Geometry check sheet. Reference: the model listing, model coordinates, mm. Round coordinates to 2 decimals unless told otherwise and drop trailing zeros. Write each loop counter-clockwise with the first axis right and the second up, starting at its lowest first coordinate (ties: lowest second). Pieces come first, ordered by that corner, then holes. Notation, with made-up numbers: (86, 33) -> (92, 33) arc R24 ccw to (92, 63) -> close; hole circle Ø8 at (64.25, 59.25). An arc over 180 degrees is marked (long way). Put each result on its own line as item: value. Start each with the question number.
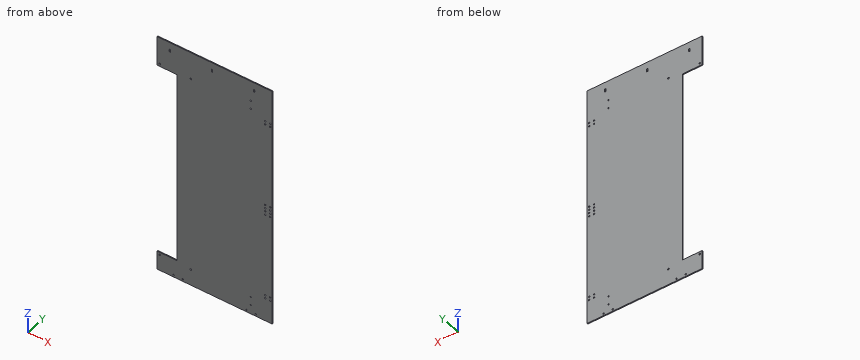
from build123d import *

# Parameters (mm, degrees)
SKETCH_1_W          = 350
SKETCH_1_H          = 3
EXTRUDE_1_DEPTH     = 725
SKETCH_2_R          = 2.6
SKETCH_2_R_2        = 2.25
SKETCH_2_R_3        = 2.05
SKETCH_2_W          = 60
SKETCH_2_H          = 580
CUT_EXTRUDE_1_DEPTH = 10


with BuildPart() as part:
    # 草图1 → 凸台-拉伸1 (new body)
    with BuildSketch(Plane.XY):
        with Locations((156.473684211, 4.735473664)):
            Rectangle(SKETCH_1_W, SKETCH_1_H)
    extrude(amount=EXTRUDE_1_DEPTH)

    # 草图2 → 切除-拉伸1 (cut)
    with BuildSketch(Plane(origin=(0, 6.235473664, 0), x_dir=(1, 0, 0), z_dir=(0, 1, 0))):
        with Locations((-11.026315789, -48.5)):
            Circle(SKETCH_2_R)
        with Locations((83.973684211, -48.5)):
            Circle(SKETCH_2_R)
        with Locations((-11.026315789, -643.5)):
            Circle(SKETCH_2_R)
        with Locations((83.973684211, -643.5)):
            Circle(SKETCH_2_R)
        with Locations((325.473684211, -341)):
            Circle(SKETCH_2_R_2)
        with Locations((310.473684211, -341)):
            Circle(SKETCH_2_R_2)
        with Locations((310.473684211, -331)):
            Circle(SKETCH_2_R_2)
        with Locations((325.473684211, -331)):
            Circle(SKETCH_2_R_2)
        with Locations((310.473684211, -80)):
            Circle(SKETCH_2_R_2)
        with Locations((310.473684211, -70)):
            Circle(SKETCH_2_R_2)
        with Locations((325.473684211, -70)):
            Circle(SKETCH_2_R_2)
        with Locations((325.473684211, -80)):
            Circle(SKETCH_2_R_2)
        with Locations((281.473684211, -6)):
            Circle(SKETCH_2_R_2)
        with Locations((253.473684211, -6)):
            Circle(SKETCH_2_R_2)
        with Locations((31.473684211, -6)):
            Circle(SKETCH_2_R_2)
        with Locations((59.473684211, -6)):
            Circle(SKETCH_2_R_2)
        with Locations((325.473684211, -351)):
            Circle(SKETCH_2_R_2)
        with Locations((310.473684211, -351)):
            Circle(SKETCH_2_R_2)
        with Locations((325.473684211, -361)):
            Circle(SKETCH_2_R_2)
        with Locations((310.473684211, -361)):
            Circle(SKETCH_2_R_2)
        with Locations((310.473684211, -612)):
            Circle(SKETCH_2_R_2)
        with Locations((325.473684211, -612)):
            Circle(SKETCH_2_R_2)
        with Locations((325.473684211, -622)):
            Circle(SKETCH_2_R_2)
        with Locations((310.473684211, -622)):
            Circle(SKETCH_2_R_2)
        with Locations((266.473684211, -639.5)):
            Circle(SKETCH_2_R_3)
        with Locations((266.473684211, -664.5)):
            Circle(SKETCH_2_R_3)
        with Locations((266.473684211, -52.5)):
            Circle(SKETCH_2_R_3)
        with Locations((266.473684211, -27.5)):
            Circle(SKETCH_2_R_3)
        with Locations((11.473684211, -346)):
            Rectangle(SKETCH_2_W, SKETCH_2_H)
        with BuildLine():
            Line((18.223684211, -702.5), (18.223684211, -697.5))
            ThreePointArc((18.223684211, -697.5), (20.473684211, -695.25), (22.723684211, -697.5))
            Line((22.723684211, -697.5), (22.723684211, -702.5))
            ThreePointArc((22.723684211, -702.5), (20.473684211, -704.75), (18.223684211, -702.5))
        make_face()
        with BuildLine():
            Line((150.723684211, -702.5), (150.723684211, -697.5))
            ThreePointArc((150.723684211, -697.5), (148.473684211, -695.25), (146.223684211, -697.5))
            Line((146.223684211, -697.5), (146.223684211, -702.5))
            ThreePointArc((146.223684211, -702.5), (148.473684211, -704.75), (150.723684211, -702.5))
        make_face()
        with BuildLine():
            Line((278.723684211, -702.5), (278.723684211, -697.5))
            ThreePointArc((278.723684211, -697.5), (276.473684211, -695.25), (274.223684211, -697.5))
            Line((274.223684211, -697.5), (274.223684211, -702.5))
            ThreePointArc((274.223684211, -702.5), (276.473684211, -704.75), (278.723684211, -702.5))
        make_face()
    extrude(amount=-CUT_EXTRUDE_1_DEPTH, mode=Mode.SUBTRACT)


solid = part.part
(1) Sectioned sample at A-A (y = 4.55). State how many separate pieces and enclosed holes the cut face has, and give its area (3 significant figures).
(2) Sectioned sample at B-B (z = 469.5). Record the cut outline in (x, y), and give its area (3 significant figures).
(3) Material ranges on L1, parallel to X at y = 5.05, z = 331; L2, parallel to X at y = 4.35, z = 6; L3, parallel to X at y = 4.1, z = 48.5, recorded low to high. Write a range as from..to.
Found:
1. separate pieces: 1
1. enclosed holes: 31
1. area: 218,000 mm2
2. outline: (41.47, 3.24) -> (331.47, 3.24) -> (331.47, 6.24) -> (41.47, 6.24) -> close
2. area: 870 mm2
3. L1: 41.47..308.22, 312.72..323.22, 327.72..331.47
3. L2: -18.53..29.22, 33.72..57.22, 61.72..251.22, 255.72..279.22, 283.72..331.47
3. L3: -18.53..-13.63, -8.43..81.37, 86.57..331.47
